Can you work these out from the drawing? Everything is in mm from the part's minimum corner. Round coordinates to 2 decimals unless told otherwise and drop trailing zeros. Loops run counter-clockwise (first coordinate to the right, second up) from the corner with the lowest first, then second, coordinate; pieces in that order, holes last. Notation, with made-up numbers: (-7, -20.5) - (4, -20.5) arc R23 cw to (4, 10.5) - close; hole circle Ø1 at (-37.5, -17.75). An arc over 180 degrees is marked (long way). Put each result on its own line as item: value. Start each with the question number.
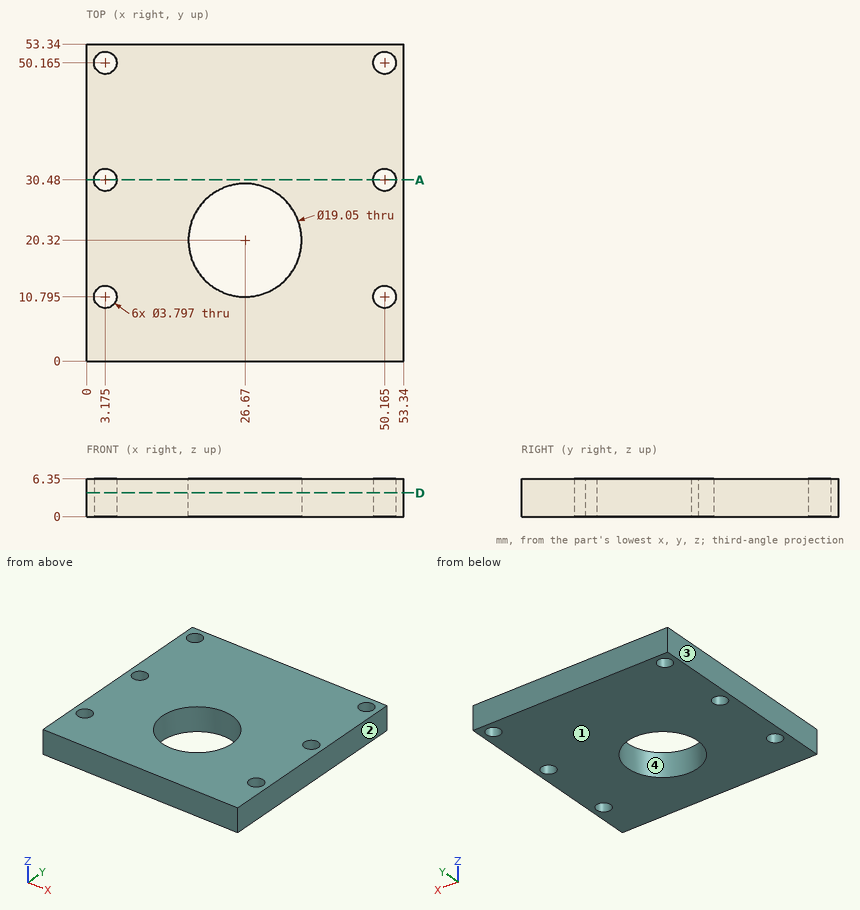
Item 1: I need wall thicknesses on line 1 (X direction, y = 30.5, z = 4.75); line 2 (Y direction, x = 26.67, z = 3.25) (1 decimal); line 3 (Y direction, x = 23.5, z = 5). Which ranges of each line are inside material? Lowest first, please. Write a range as from..to.
Item 2: Suppose I cut it at D-D, the plane z = 4. Count the separate pieces of the cut face and the enclosed holes in it, then the cut area to 3 significant figures.
Item 3: Thinking about a two-plate mould opening in X: for the marked faces 1, 2, 3 and 4, which applies, released by +X, released by -X, zero draft, split by the parting line, or undercut?
Item 4: Suppose I cut it at A-A, the plane y = 30.48. List the corners of the cut face in (x, z) for me.
Numbers:
1. line 1: 0..1.28, 5.07..48.27, 52.06..53.34
1. line 2: 0..10.8, 29.8..53.3
1. line 3: 0..11.34, 29.3..53.34
2. separate pieces: 1
2. enclosed holes: 7
2. area: 2,490 mm^2
3. face 1: zero draft
3. face 2: released by +X
3. face 3: released by -X
3. face 4: undercut
4. outline: (0, 0) - (1.28, 0) - (1.28, 6.35) - (0, 6.35) - close; (5.07, 0) - (48.27, 0) - (48.27, 6.35) - (5.07, 6.35) - close; (52.06, 0) - (53.34, 0) - (53.34, 6.35) - (52.06, 6.35) - close
